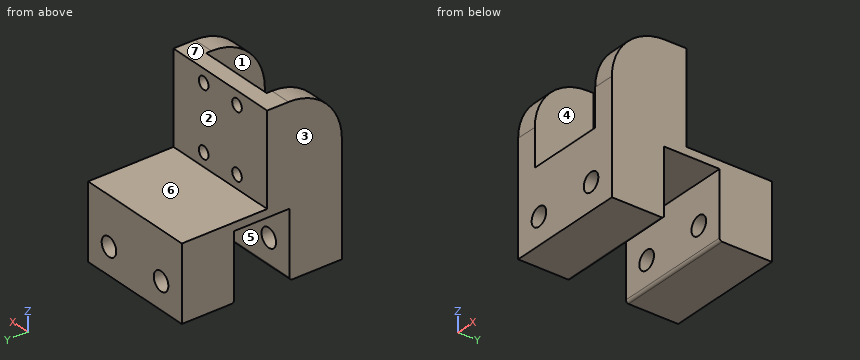
from build123d import *

# Parameters (mm, degrees)
SKETCH_1_W          = 22.5
SKETCH_1_H          = 17
EXTRUDE_1_DEPTH     = 3
HOLE_WIZARD_1_D     = 2.3
SKETCH_5_W          = 22.5
SKETCH_5_H          = 4
SKETCH_5_H_2        = 3
EXTRUDE_2_DEPTH     = 1.5
SKETCH_8_W          = 22.5
SKETCH_8_H          = 10
EXTRUDE_3_DEPTH     = 1.5
SKETCH_9_W          = 17
SKETCH_9_H          = 14
EXTRUDE_4_DEPTH     = 4
SKETCH_10_W         = 17
SKETCH_10_H         = 14
EXTRUDE_5_DEPTH     = 4
SKETCH_11_W         = 22.5
SKETCH_11_H         = 11
EXTRUDE_6_DEPTH     = 1.5
HOLE_WIZARD_3_D     = 3.3
SKETCH_18_W         = 22.5
SKETCH_18_H         = 10
EXTRUDE_7_DEPTH     = 2.4
SKETCH_21_W         = 22.5
SKETCH_21_H         = 3
EXTRUDE_8_DEPTH     = 2.4
SKETCH_22_W         = 22.5
SKETCH_22_H         = 8
EXTRUDE_9_DEPTH     = 2.4
SKETCH_25_W         = 22.5
SKETCH_25_H         = 8
SKETCH_25_H_2       = 3
CUT_EXTRUDE_1_DEPTH = 36.949582751
SKETCH_26_W         = 22.5
SKETCH_26_H         = 10
EXTRUDE_10_DEPTH    = 10
FILLET_1_R          = 10
HOLE_WIZARD_4_D     = 3.5
SKETCH_30_W         = 12.4
SKETCH_30_H         = 0.2
CUT_EXTRUDE_2_DEPTH = 38.000135135
FILLET_3_R          = 0.5


with BuildPart() as part:
    # 草图1 → 凸台-拉伸1 (new body)
    with BuildSketch(Plane(origin=(0, 0, 0), x_dir=(1, 0, 0), z_dir=(0, 1, 0))):
        Rectangle(SKETCH_1_W, SKETCH_1_H)
    extrude(amount=EXTRUDE_1_DEPTH)

    # 孔1 (through all)
    with Locations(Plane(origin=(0, 3, 0), x_dir=(1, 0, 0), z_dir=(0, 1, 0))):
        with Locations((-4, 6), (4, 6), (-4, -6), (4, -6)):
            Hole(HOLE_WIZARD_1_D / 2)

    # 草图5 → 凸台-拉伸2 (add)
    with BuildSketch(Plane(origin=(0, 0, -8.5), x_dir=(-1, 0, 0), z_dir=(0, 0, -1))):
        with Locations((0, -2)):
            Rectangle(SKETCH_5_W, SKETCH_5_H)
        with Locations((0, 1.5)):
            Rectangle(SKETCH_5_W, SKETCH_5_H_2)
        with Locations((0, 4.5)):
            Rectangle(SKETCH_5_W, SKETCH_5_H_2)
    extrude(amount=EXTRUDE_2_DEPTH)

    # 草图8 → 凸台-拉伸3 (add)
    with BuildSketch(Plane(origin=(0, 0, -10), x_dir=(-1, 0, 0), z_dir=(0, 0, -1))):
        with Locations((0, -9)):
            Rectangle(SKETCH_8_W, SKETCH_8_H)
        with Locations((0, 11)):
            Rectangle(SKETCH_8_W, SKETCH_8_H)
    extrude(amount=-EXTRUDE_3_DEPTH)

    # 草图9 → 凸台-拉伸4 (add)
    with BuildSketch(Plane.ZY.offset(11.25)):
        with Locations((0, -7)):
            Rectangle(SKETCH_9_W, SKETCH_9_H)
    extrude(amount=-EXTRUDE_4_DEPTH)

    # 草图10 → 凸台-拉伸5 (add)
    with BuildSketch(Plane(origin=(11.25, 0, 0), x_dir=(0, 0, -1), z_dir=(1, 0, 0))):
        with Locations((0, -7)):
            Rectangle(SKETCH_10_W, SKETCH_10_H)
    extrude(amount=-EXTRUDE_5_DEPTH)

    # 草图11 → 凸台-拉伸6 (add)
    with BuildSketch(Plane(origin=(0, 0, -10), x_dir=(-1, 0, 0), z_dir=(0, 0, -1))):
        with Locations((0, 21.5)):
            Rectangle(SKETCH_11_W, SKETCH_11_H)
    extrude(amount=-EXTRUDE_6_DEPTH)

    # 孔3 (through all)
    with Locations(Plane(origin=(0, 0, -10), x_dir=(-1, 0, 0), z_dir=(0, 0, -1))):
        with Locations((-7.25, 22), (7.25, 22)):
            Hole(HOLE_WIZARD_3_D / 2)

    # 草图18 → 凸台-拉伸7 (add)
    with BuildSketch(Plane(origin=(0, 0, -10), x_dir=(-1, 0, 0), z_dir=(0, 0, -1))):
        with Locations((0, -9)):
            Rectangle(SKETCH_18_W, SKETCH_18_H)
        with Locations((0, 22)):
            Rectangle(SKETCH_18_W, SKETCH_18_H)
    extrude(amount=EXTRUDE_7_DEPTH)

    # 草图21 → 凸台-拉伸8 (add)
    with BuildSketch(Plane(origin=(0, 0, -10), x_dir=(-1, 0, 0), z_dir=(0, 0, -1))):
        with Locations((0, -2.5)):
            Rectangle(SKETCH_21_W, SKETCH_21_H)
    extrude(amount=EXTRUDE_8_DEPTH)

    # 草图22 → 凸台-拉伸9 (add)
    with BuildSketch(Plane(origin=(0, 0, -10), x_dir=(-1, 0, 0), z_dir=(0, 0, -1))):
        with Locations((0, 13)):
            Rectangle(SKETCH_22_W, SKETCH_22_H)
    extrude(amount=EXTRUDE_9_DEPTH)

    # 草图25 → 切除-拉伸1 (cut, through all)
    with BuildSketch(Plane(origin=(0, 0, -12.4), x_dir=(-1, 0, 0), z_dir=(0, 0, -1))):
        with Locations((0, 23)):
            Rectangle(SKETCH_25_W, SKETCH_25_H)
        with Locations((0, -12.5)):
            Rectangle(SKETCH_25_W, SKETCH_25_H_2)
    extrude(amount=-CUT_EXTRUDE_1_DEPTH, mode=Mode.SUBTRACT)

    # 草图26 → 凸台-拉伸10 (add)
    with BuildSketch(Plane(origin=(0, 0, -12.4), x_dir=(-1, 0, 0), z_dir=(0, 0, -1))):
        with Locations((0, 14)):
            Rectangle(SKETCH_26_W, SKETCH_26_H)
        with Locations((0, -6)):
            Rectangle(SKETCH_26_W, SKETCH_26_H)
    extrude(amount=EXTRUDE_10_DEPTH)

    # 圆角1
    fillet_1_edges = [part.edges().sort_by_distance(p)[0] for p in [
        (-9.25, -11, 8.5),
        (9.25, -11, 8.5),
    ]]
    fillet(fillet_1_edges, radius=FILLET_1_R)

    # 孔4 (through all)
    with Locations(Plane(origin=(0, 19, 0), x_dir=(1, 0, 0), z_dir=(0, 1, 0))):
        with Locations((-6.25, 17.4), (6.25, 17.4)):
            Hole(HOLE_WIZARD_4_D / 2)

    # 草图30 → 切除-拉伸2 (cut, through all)
    with BuildSketch(Plane(origin=(11.25, 0, 0), x_dir=(0, 0, -1), z_dir=(1, 0, 0))):
        with Locations((16.2, 9.1)):
            Rectangle(SKETCH_30_W, SKETCH_30_H)
        with Locations((16.2, -1.1)):
            Rectangle(SKETCH_30_W, SKETCH_30_H)
    extrude(amount=-CUT_EXTRUDE_2_DEPTH, mode=Mode.SUBTRACT)

    # 圆角3
    fillet_3_edges = [part.edges().sort_by_distance(p)[0] for p in [
        (0, 9.2, -22.4),
        (0, -1.2, -22.4),
    ]]
    fillet(fillet_3_edges, radius=FILLET_3_R)


solid = part.part
Can you work these out from the model? Positions are in its coordinate system, mm. Face numbers are marked on the shaded views. A direction names the side the tool comes from. Coordinates: 2 decimals unless noted, no trailing zeros. Order: outer loops, then holes, each group sorted by start corner. A loop starts at its lowest first (then second) coordinate and runs counter-clockwise, first axis right, second up. Notation, with made-up numbers: (42.5, 35.5) -> (68.5, 35.5) arc R16 cw to (68.5, 49.5) -> close; hole circle Ø4 at (25, 56). An arc over 180 degrees is marked (long way). Use one line per item in the form item = value.
Q1. Imagine slicing it at B-B, the plane z = -6. List the corners of the cut face in (x, y) for me, then the cut area to 3 significant figures.
From the geometry:
outline = (-11.25, -11) -> (-7.25, -11) -> (-7.25, 0) -> (-5.15, 0) -> (-5.15, 3) -> (-11.25, 3) -> close; (-2.85, 0) -> (2.85, 0) -> (2.85, 3) -> (-2.85, 3) -> close; (5.15, 0) -> (7.25, 0) -> (7.25, -11) -> (11.25, -11) -> (11.25, 3) -> (5.15, 3) -> close
area = 142 mm²
Q2. Imagine slicing it at D-D, the plane y = 15.25. List the corners of the cut face in (x, z) for me, then the cut area to 3 significant figures.
From the geometry:
outline = (-11.25, -22.4) -> (11.25, -22.4) -> (11.25, -8.5) -> (-11.25, -8.5) -> close; hole circle Ø3.5 at (-6.25, -17.4); hole circle Ø3.5 at (6.25, -17.4)
area = 294 mm²
Q3. We'd pull the mould along X, two halves only. Please class the marked faces 1, 2, 3 and 4: released by +X, released by -X, zero draft, split by the parting line, or undercut.
From the geometry:
face_1 = undercut
face_2 = zero draft
face_3 = released by -X
face_4 = undercut
Q4. Imagine slicing it at A-A, the plane z = -17.4. List the corners of the cut face in (x, y) for me, then the cut area to 3 significant figures.
From the geometry:
outline = (-11.25, -11) -> (-8, -11) -> (-8, -1.2) -> (-11.25, -1.2) -> close; (-11.25, 9.2) -> (-8, 9.2) -> (-8, 19) -> (-11.25, 19) -> close; (-4.5, -11) -> (4.5, -11) -> (4.5, -1.2) -> (-4.5, -1.2) -> close; (-4.5, 9.2) -> (4.5, 9.2) -> (4.5, 19) -> (-4.5, 19) -> close; (8, -11) -> (11.25, -11) -> (11.25, -1.2) -> (8, -1.2) -> close; (8, 9.2) -> (11.25, 9.2) -> (11.25, 19) -> (8, 19) -> close
area = 304 mm²
Q5. I need wall thicknesses on L1, parallel to Z at x = -4, y = 1.05; L2, parallel to X at y = -5.5, z = -4.5; L3, parallel to Y at x = -2.25, z = -17.5. Which ranges of each line are inside material? Lowest first, please.
From the geometry:
L1 = -10 to -7.15, -4.85 to 4.85, 7.15 to 8.5
L2 = -11.25 to -7.25, 7.25 to 11.25
L3 = -11 to -1.2, 9.2 to 19
Q6. Imagine slicing it at C-C, the plane x = 6.25. List the corners of the cut face in (y, z) for me, then the cut area to 3 significant figures.
From the geometry:
outline = (-11, -22.4) -> (-1.7, -22.4) arc R0.5 ccw to (-1.2, -21.9) -> (-1.2, -19.15) -> (-11, -19.15) -> close; (-11, -15.65) -> (-1.2, -15.65) -> (-1.2, -10) -> (9.2, -10) -> (9.2, -15.65) -> (19, -15.65) -> (19, -8.5) -> (3, -8.5) -> (3, 8.5) -> (0, 8.5) -> (0, -8.5) -> (-11, -8.5) -> close; (9.2, -21.9) arc R0.5 ccw to (9.7, -22.4) -> (19, -22.4) -> (19, -19.15) -> (9.2, -19.15) -> close
area = 270 mm²
Q7. Will these pins go through, and if not, where does the flat tip stop? P1, Ø11.5, axis at x = -1, y = 4.5, coming from the -Z side; P2, Ø3, axis at x = -4, z = 6, coming from the -Y side; P3, Ø5, axis at x = 3, y = 1.5, coming from the -Z side; P4, Ø8, axis at x = -1, y = 11, coming from the +Z side.
From the geometry:
P1 = -22.4
P2 = 0
P3 = -10
P4 = -8.5
Q8. Which directions (+Z, -Z, +X, -X, +Y, -Y) give clear straight access to the entire face, cutting with the end or side of a thin tool? Please do the marked faces 5, 6 and 7.
From the geometry:
face_5 = -Z, +X, -X
face_6 = +Z, +X, -X, +Y
face_7 = +Z, +X, -X, +Y, -Y
